Here's the drawing with two shaded views (mm, measured from the low corner). I have some questions. A direction names the side the tool comes from. Round coordinates to 2 decimals unless told otherwise and drop trailing zeros. Order: outer loops, then holes, each group sorted by start corner. A loop starts at its lowest first (then second) coordinate and runs counter-clockwise, first axis right, second up. Notation, with made-up numbers: (15.25, 75) -> (52.25, 75) arc R29 ccw to (52.25, 101) -> close; hole circle Ø10 at (-38, 69.25). An arc over 180 degrees is marked (long way). Put each result on its own line as item: value. Start each with the question number.
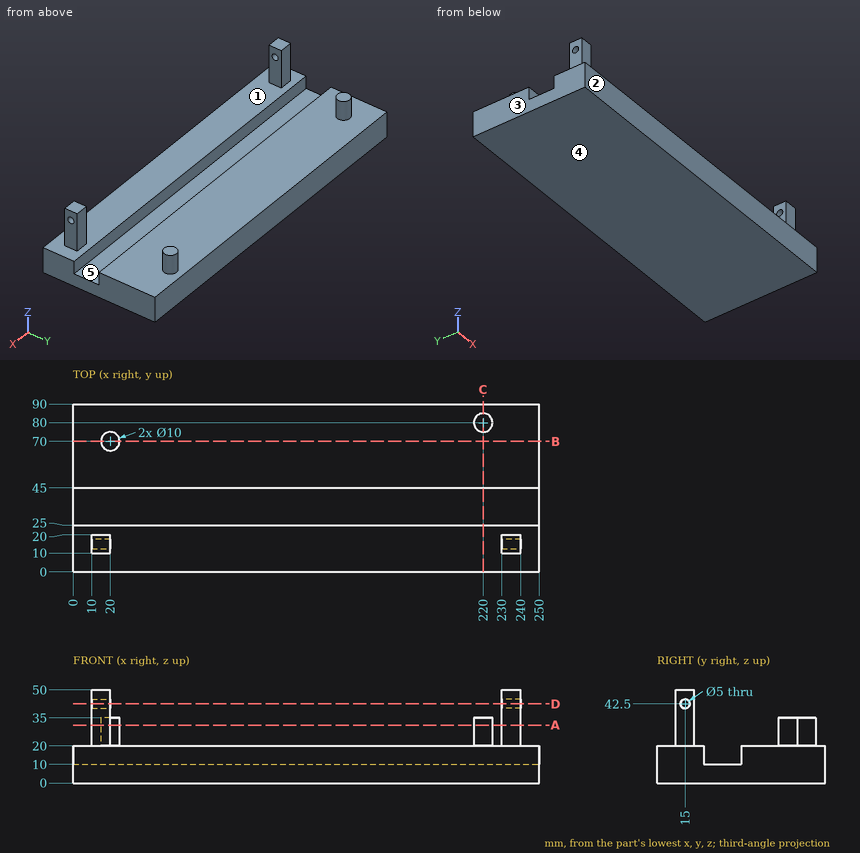
1. For pin 1 Ø11 at (x, z) = (16, 38) entering from -Y; pin 2 Ø5 at (y, z) = (16.5, 36.5) entering from +X; pin 3 Ø22.5 at (x, y) = (159.5, 58) entering from +Z, each with a flat end and sliding along its axis, tell me the tip position at first contact or that it passes through.
2. If we section it at D-D, the plane z = 42.5: Please give me the cut outline in (x, y).
3. Thinking about a two-plate mould opening in X: for the marked faces 1, 2 and 3, which applies, +X half, -X half, draft (parallel to the pull), parting line (faces both ways), or undercut?
4. If we section it at A-A, the plane z = 31: Please give me the cut outline in (x, y), then the cut area to 3 significant figures.
5. Which directions (+Z, -Z, +X, -X, +Y, -Y) give clear straight access to the entire face, cutting with the end or side of a thin tool? Please do the marked faces 4 and 5.
6. I need wall thicknesses on L1, parallel to Y at x = 234, z = 42; L2, parallel to Z at x = 16, y = 15; L3, parallel to Z at x = 172, y = 83. Which ranges of each line are inside material? Lowest first, please.
7. If we section it at B-B, the plane y = 70: Please give me the cut outline in (x, z), then the cut area to 3 significant figures.
8. If we section it at C-C, the plane x = 220: Please give me the cut outline in (y, z).
Results below:
1. pin 1: y = 10
1. pin 2: x = 240
1. pin 3: z = 20
2. outline: (10, 10) -> (20, 10) -> (20, 12.5) -> (10, 12.5) -> close; (10, 17.5) -> (20, 17.5) -> (20, 20) -> (10, 20) -> close; (230, 10) -> (240, 10) -> (240, 12.5) -> (230, 12.5) -> close; (230, 17.5) -> (240, 17.5) -> (240, 20) -> (230, 20) -> close
3. face 1: undercut
3. face 2: draft
3. face 3: -X half
4. outline: (10, 10) -> (20, 10) -> (20, 20) -> (10, 20) -> close; circle Ø10 at (20, 70); circle Ø10 at (220, 80); (230, 10) -> (240, 10) -> (240, 20) -> (230, 20) -> close
4. area: 357 mm2
5. face 4: -Z, +X, -X, +Y, -Y
5. face 5: +Z, +X, -X
6. L1: 10 to 12.55, 17.45 to 20
6. L2: 0 to 40, 45 to 50
6. L3: 0 to 20
7. outline: (0, 0) -> (250, 0) -> (250, 20) -> (25, 20) -> (25, 35) -> (15, 35) -> (15, 20) -> (0, 20) -> close
7. area: 5,150 mm2
8. outline: (0, 0) -> (90, 0) -> (90, 20) -> (85, 20) -> (85, 35) -> (75, 35) -> (75, 20) -> (45, 20) -> (45, 10) -> (25, 10) -> (25, 20) -> (0, 20) -> close
